from build123d import *

# Parameters (mm, degrees)
SCALE1_SCALE = 0.5


with BuildPart() as part:
    # Sketch1 → Revolve1 (revolve)
    with BuildSketch(Plane.XY):
        with BuildLine():
            Line((0, 0), (60, 0))
            ThreePointArc((60, 0), (77.5, 4.689110868), (90.310889132, 17.5))
            Line((90.310889132, 17.5), (121.791448663, 72.025928557))
            ThreePointArc((121.791448663, 72.025928557), (124.472789107, 74.805615606), (128.143930379, 76.005185711))
            ThreePointArc((128.143930379, 76.005185711), (129.994814289, 78.143930379), (127.856069621, 79.994814289))
            ThreePointArc((127.856069621, 79.994814289), (122.349357715, 78.19545913), (118.327347047, 74.025928557))
            Line((118.327347047, 74.025928557), (86.846787517, 19.5))
            ThreePointArc((86.846787517, 19.5), (75.5, 8.153212483), (60, 4))
            Line((60, 4), (0, 4))
            Line((0, 4), (0, 0))
        make_face()
    revolve(axis=Axis((0, 4, 0), (0, -1, 0)))


with BuildPart() as part_1:
    # Scale1: scaled about (0, 35.690345414, 0)
    add(part.part.scale(SCALE1_SCALE).moved(Location((0, 17.845172707, 0))))


solid = part_1.part
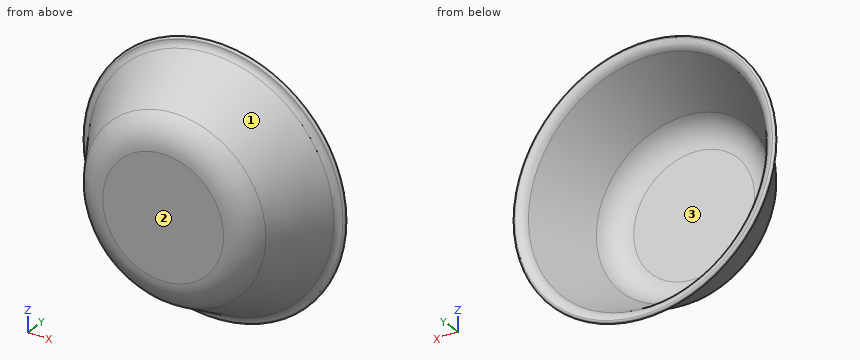
Here's how the part is built. I have some questions about the finished solid (model axes, mm). Face numbers are marked on the shaded views. Round coordinates to 2 decimals unless told otherwise and drop trailing zeros. Loops run counter-clockwise (first coordinate to the right, second up) from the corner with the lowest first, then second, coordinate; pieces in that order, holes last.
1. We'd pull the mould along Z, two halves only. Please class the marked faces 1, 2 and 3: +Z half, -Z half, draft (parallel to the pull), parting line (faces both ways), or undercut.
Answer list:
face 1: parting line
face 2: draft
face 3: undercut
2. If we section it at A-A on x = 0: Write out the boundary of the cut face in (y, z), plus the area to 3 significant figures.
Answer list:
outline: (17.85, -30) arc R17.5 ccw to (26.6, -45.16) - (53.86, -60.9) arc R4 cw to (55.85, -64.07) arc R1 ccw to (57.84, -63.93) arc R6 ccw to (54.86, -59.16) - (27.6, -43.42) arc R15.5 cw to (19.85, -30) - (19.85, 30) arc R15.5 cw to (27.6, 43.42) - (54.86, 59.16) arc R6 ccw to (57.84, 63.93) arc R1 ccw to (55.85, 64.07) arc R4 cw to (53.86, 60.9) - (26.6, 45.16) arc R17.5 ccw to (17.85, 30) - close
area: 338 mm2
3. For P1, Ø12, axis at y = 38, z = -26.5, coming from the -X side; P2, Ø1, axis at y = 40, z = -12.5, coming from the -X side; P3, Ø1.5, axis at y = 43, z = 21, coming from the +X side, each with a flat end and sliding along its axis, tell me the tip position at first contact or that it passes through.
Answer list:
P1: stops at x = -49.47
P2: stops at x = -51.72
P3: stops at x = 50.99
4. If I drill on line 1 along X through (y, z) = (25.5, -4); line 2 along Z through (x, y) = (50, 45); line 3 along X through (y, z) = (54.5, -14.5), over which ranges is the centre line in solid material (lowest first)?
Answer list:
line 1: x = -44.29 to -41.78, 41.78 to 44.29
line 2: z = -24.73 to -18.95, 18.95 to 24.73
line 3: x = -59.62 to -57.15, 57.15 to 59.62
5. If we section it at C-C on y = 40: Write out the boundary of the cut face in (x, z).
Answer list:
outline: circle Ø105.79 at (0, 0); hole circle Ø101.17 at (0, 0)
6. If we section it at B-B on z = 0: Write out the boundary of the cut face in (x, y).
Answer list:
outline: (-64.07, 55.85) arc R4 cw to (-60.9, 53.86) - (-45.16, 26.6) arc R17.5 ccw to (-30, 17.85) - (30, 17.85) arc R17.5 ccw to (45.16, 26.6) - (60.9, 53.86) arc R4 cw to (64.07, 55.85) arc R1 ccw to (63.93, 57.84) arc R6 ccw to (59.16, 54.86) - (43.42, 27.6) arc R15.5 cw to (30, 19.85) - (-30, 19.85) arc R15.5 cw to (-43.42, 27.6) - (-59.16, 54.86) arc R6 ccw to (-63.93, 57.84) arc R1 ccw to start
